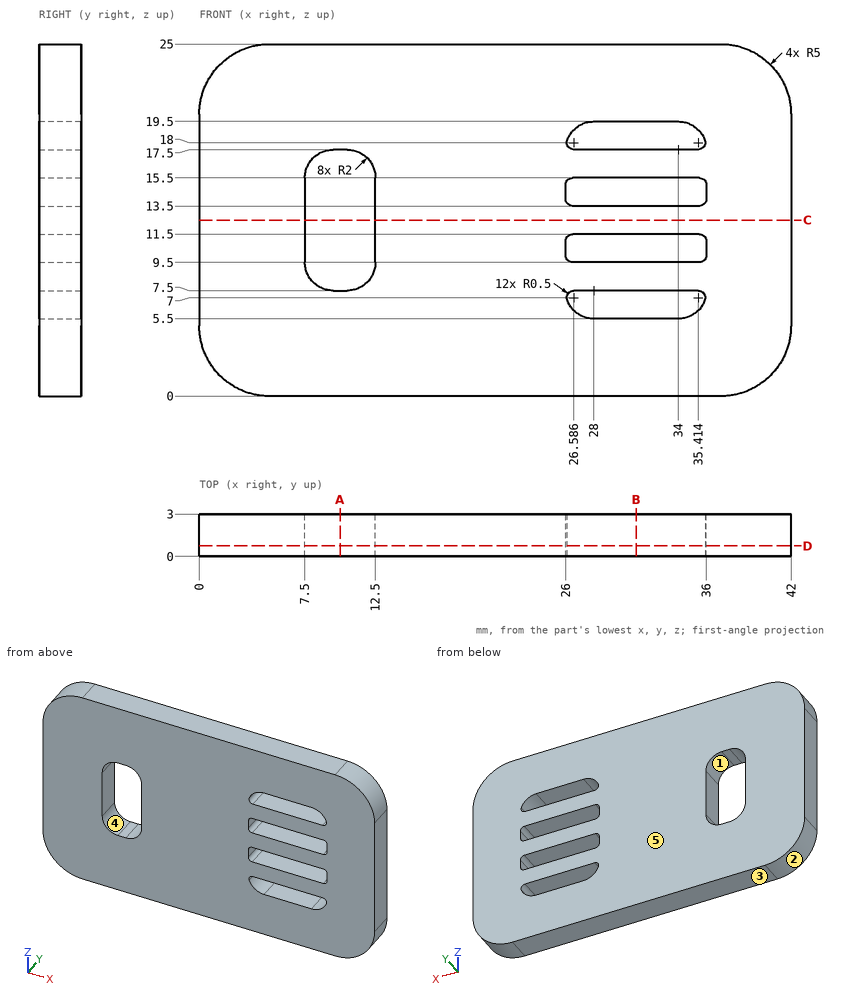
Drawing for the job (mm, zero at the part's lowest x, y, z). A direction names the side the tool comes from. Give positions to 0.01 mm unless a question says otherwise; leave off trailing zeros. Loops run counter-clockwise (first coordinate to the right, second up) from the corner with the lowest first, then second, coordinate; pieces in that order, holes last. Notation, with made-up numbers: M 71,-20.5 L 98,-20.5 A12 cw 98,-16.5 Z; hole C 12,46 d8. An arc over 180 degrees is marked long. One line per question, with ' | ' between items. Start each with the question number.
1. Saw through at D-D on y = 0.75. State how many separate pieces and enclosed holes the cut face has, plus the area to 3 significant figures.
2. 3-axis set-ups, long thin cutter, end or side, ignore diameter. For the marked faces 4 and 5: which of +Z, -Z, +X, -X, +Y, -Y reach the whole face in a straight line?
3. Probe L1, parallel to Z at x = 32.5, y = 1; L2, parallel to Z at x = 27, y = 1.45; L3, parallel to X at y = 2.05, z = 12. List the from-to ranges inside material, lowest first. Write a range as from..to.
4. Saw through at B-B on x = 31. Give the cut face in (y, z), plus the area to 3 significant figures.
5. Saw through at A-A on x = 10. Give the cut face in (y, z).
6. Saw through at C-C on z = 12.5. Give the cut face in (x, y).
7. Two-plate mould, pull along X, no slides. Class the marked faces 1, 2 and 3: pulls with the +X half, pulls with the -X half, needs draft (parallel to the pull), parting line crosses it, or undercut.
Result sheet:
1) separate pieces: 1 | enclosed holes: 5 | area: 906 mm^2
2) face 4: +Y, -Y | face 5: +Z, -Z, +X, -X, +Y
3) L1: z = 0..5.5, 7.5..9.5, 11.5..13.5, 15.5..17.5, 19.5..25 | L2: z = 0..5.77, 7.5..9.5, 11.5..13.5, 15.5..17.5, 19.23..25 | L3: x = 0..7.5, 12.5..42
4) outline: M 0,0 L 3,0 L 3,5.5 L 0,5.5 Z; M 0,7.5 L 3,7.5 L 3,9.5 L 0,9.5 Z; M 0,11.5 L 3,11.5 L 3,13.5 L 0,13.5 Z; M 0,15.5 L 3,15.5 L 3,17.5 L 0,17.5 Z; M 0,19.5 L 3,19.5 L 3,25 L 0,25 Z | area: 51.0 mm^2
5) outline: M 0,0 L 3,0 L 3,7.5 L 0,7.5 Z; M 0,17.5 L 3,17.5 L 3,25 L 0,25 Z
6) outline: M 0,0 L 7.5,0 L 7.5,3 L 0,3 Z; M 12.5,0 L 42,0 L 42,3 L 12.5,3 Z
7) face 1: undercut | face 2: pulls with the -X half | face 3: needs draft
